```python
from build123d import *

# Parameters (mm, degrees)
SKETCH2_R           = 10
SKETCH2_R_2         = 6.5
BOSS_EXTRUDE1_DEPTH = 2
SKETCH1_R           = 8.5
SKETCH4_R           = 6.5
CUT_EXTRUDE1_DEPTH  = 16.000000167


with BuildPart() as part:
    # Sketch2 → Boss-Extrude1 (new body)
    with BuildSketch(Plane(origin=(0, -5, 0), x_dir=(1, 0, 0), z_dir=(0, 1, 0))):
        with Locations(Location((0, 0, 0), (0, 0, 270))):
            Circle(SKETCH2_R)
        with Locations(Location((0, 0, 0), (0, 0, 270))):
            Circle(SKETCH2_R_2, mode=Mode.SUBTRACT)
    extrude(amount=-BOSS_EXTRUDE1_DEPTH)

    # Sketch1 → section 1 of loft6
    with BuildSketch(Plane(origin=(0, 0, 0), x_dir=(1, 0, 0), z_dir=(0, 1, 0)), mode=Mode.PRIVATE) as loft6_s1:
        Circle(SKETCH1_R)
    # loft up to a face of the part (loft6)
    loft([Face(Wire([part.edges().sort_by_distance((7.289686274, -5, -6.845471059))[0]])), loft6_s1.sketch])

    # Sketch4 → Cut-Extrude1 (cut, through all)
    with BuildSketch(Plane.XZ.offset(5)):
        with Locations(Location((0, 0, 0), (0, 0, 90))):
            Circle(SKETCH4_R)
    extrude(amount=-CUT_EXTRUDE1_DEPTH, mode=Mode.SUBTRACT)


solid = part.part
```
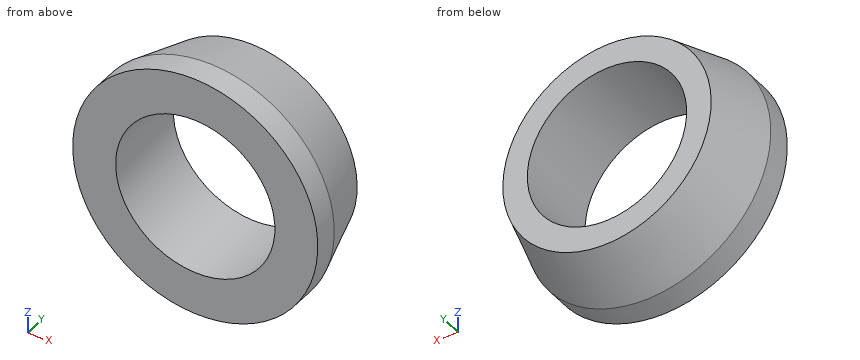
Geometry: final body of the model. Coordinates: model frame, mm. Round coordinates to 2 decimals unless told otherwise and drop trailing zeros. Loops run counter-clockwise (first coordinate to the right, second up) from the corner with the lowest first, then second, coordinate; pieces in that order, holes last.
Item 1: Section C-C, the plane y = -2.5. Output: boundary loops of the cut face in (x, z), plus the area to 3 significant figures.
Checked values:
outline: circle Ø18.5 at (0, 0); hole circle Ø13 at (0, 0)
area: 136 mm2
Item 2: Section A-A, the plane z = 0. Output: boundary loops of the cut face in (x, y).
Checked values:
outline: (-10, -7) - (-6.5, -7) - (-6.5, 0) - (-8.5, 0) - (-10, -5) - close; (6.5, -7) - (10, -7) - (10, -5) - (8.5, 0) - (6.5, 0) - close
Item 3: Section B-B, the plane y = -5.5. Output: boundary loops of the cut face in (x, z).
Checked values:
outline: circle Ø20 at (0, 0); hole circle Ø13 at (0, 0)
Item 4: Line query: L1, parallel to Z at x = -4.25, y = -0.75; L2, parallel to Z at x = 0, y = -4.5; L3, parallel to X at y = -6.5, z = -5. Output: solid intervals per line, ascending.
Checked values:
L1: z = -7.62 to -4.92, 4.92 to 7.62
L2: z = -9.85 to -6.5, 6.5 to 9.85
L3: x = -8.66 to -4.15, 4.15 to 8.66
Item 5: Contact query for flat-ended pins moving along their axis: P1, Ø8, axis at x = 0, z = 0, coming from the +Y side; P2, Ø1.5, axis at y = -2.5, z = -3.5, coming from the -X side. Output: stop coordinate, or through.
Checked values:
P1: passes through
P2: stops at x = -8.93
